Geometry check sheet. Reference: the model listing, model coordinates, mm. Coordinates: 2 decimals unless noted, no trailing zeros. Write each loop counter-clockwise with the first axis right and the second up, starting at its lowest first coordinate (ties: lowest second). Pieces come first, ordered by that corner, then holes. Notation, with made-up numbers: (45, 16) -> (101, 16) arc R23 cw to (101, 42) -> close; hole circle Ø3 at (65, -19.5). An arc over 180 degrees is marked (long way). Answer as CSV lines item,"result".
```python
from build123d import *

# Parameters (mm, degrees)
F0_R     = 50.8
F1_DEPTH = 6.35
F2_D     = 13.208


with BuildPart() as f1:
    # F0 (on Front) → F1 (new body)
    with BuildSketch(Plane.XZ):
        Circle(F0_R)
    extrude(amount=F1_DEPTH)

    # F2 (through all)
    with Locations(Plane(origin=(0, 0, 0), x_dir=(1, 0, 0), z_dir=(0, 1, 0))):
        with Locations((0, 0)):
            Hole(F2_D / 2)

    # F3 (on Top) → F4 (revolve)
    with BuildSketch(Plane.XY):
        Polygon((50.8, 0), (50.8, -6.35), (56.299261, -3.175), align=None)
    revolve(axis=Axis((0, -6.35, 0), (0, -1, 0)))


solid = f1.part
```
Item 1: Cross-section at A-A, the plane x = 0. Record the cut outline in (y, z) (3 decimals).
Responses:
outline,"(-6.35, -50.8) -> (-3.175, -56.299) -> (0, -50.8) -> (0, -6.604) -> (-6.35, -6.604) -> close; (-6.35, 6.604) -> (0, 6.604) -> (0, 50.8) -> (-3.175, 56.299) -> (-6.35, 50.8) -> close"
Item 2: Cross-section at B-B, the plane z = 0. Record the cut outline in (x, y) (3 decimals).
Responses:
outline,"(-56.299, -3.175) -> (-50.8, -6.35) -> (-6.604, -6.35) -> (-6.604, 0) -> (-50.8, 0) -> close; (6.604, -6.35) -> (50.8, -6.35) -> (56.299, -3.175) -> (50.8, 0) -> (6.604, 0) -> close"
Item 3: Depth check by flat-ended pin: pin 1 Ø1.5 at (y, z) = (-4, 30) entering from +X; pin 2 Ø1 at (y, z) = (-4, 7.5) entering from +X. Enter the tip coordinate at first touch or a pass-through.
Responses:
pin 1,"stops at x = 47.56"
pin 2,"stops at x = 55.23"
Item 4: Thickness scan on probe 1 along Z at (x, y) = (0, -4); probe 2 along Z at (x, y) = (0, -3.5); probe 3 along Y at (x, z) = (-30, 45). Record the ranges inside material, lowest first.
Responses:
probe 1,"z = -54.87 to -6.6, 6.6 to 54.87"
probe 2,"z = -55.74 to -6.6, 6.6 to 55.74"
probe 3,"y = -4.45 to -1.9"
Item 5: Cross-section at C-C, the plane y = -1. Record the cut outline in (x, z), plus the area to 3 significant figures.
Responses:
outline,"circle Ø105.06 at (0, 0); hole circle Ø13.21 at (0, 0)"
area,"8,530 mm2"
